Autodesk Inventor part; units mm, degrees
ref_plane "YZ Plane" through (0, 0, 0) normal (1, 0, 0) x (0, 1, 0)
ref_plane "XZ Plane" through (0, 0, 0) normal (0, 1, 0) x (-1, 0, 0)
ref_plane "XY Plane" through (0, 0, 0) normal (0, 0, 1) x (1, 0, 0)
sketch "Skizze3" plane through (0, 0, 0) normal (1, 0, 0) x (0, 1, 0)
  line L0 (0, 60) -> (0, -10) construction
  line L1 (-35, 0) -> (35, 0) construction
  line L2 (25, 0) -> (25, 22.5) construction
  line L3 (25, 50) -> (-25, 50)
  line L4 (-25, 50) -> (-25, 26)
  line L5 (11.1, 0) -> (11.1, 26) construction
  line L6 (11.1, 26) -> (-11.1, 26) construction
  line L7 (-11.1, 26) -> (-11.1, 0) construction
  line L8 (11.1, 22.5) -> (25, 22.5)
  line L9 (11.1, 22.5) -> (11.1, 26)
  line L10 (11.1, 26) -> (-25, 26)
  line L11 (-25, 26) -> (-25, 0) construction
  line L12 (25, 22.5) -> (25, 50)
  point P0 (0, 0)
  dimension "d8" = 100
  dimension "d9" = 50
  dimension "d10" = 52
  dimension "d11" = 22.2
  dimension "d13" = 45
revolve "Grundkörper" add sketch "Skizze3" angle 360 about axis through (0, 0, 0) along (0, 1, 0)
sketch "Skizze4" plane through (0, 0, 0) normal (1, 0, 0) x (0, 1, 0)
  line L0 (-25, 50) -> (25, 50) construction
  line L1 (0, 48) -> (0, -8) construction
  line L2 (-15, 50) -> (-15, 30)
  line L3 (-15, 30) -> (15, 30)
  line L4 (15, 30) -> (15, 50)
  line L5 (-15, 50) -> (15, 50)
  point P0 (0, 0)
  dimension "d17" = 30
  dimension "d18" = 20
extrude "Profil_Ausschnitt" cut sketch "Skizze4" along normal through all both and the other way through all
sketch "Skizze5" plane through (0, -25, 0) normal (0, -1, 0) x (1, 0, 0)
  circle A0 centre (0, 0) radius 50 construction
  line L0 (0, 70) -> (0, -70) construction
  line L1 (-40, 30) -> (40, 30) construction
  line L2 (0, 30) -> (0, 50) construction
  point P0 (0, 40)
hole "DIN7984_M8_Boh" at (0, -25, 40) direction (0, 1, 0) diameter 9 end up to surface counterbore diameter 15 counterbore depth 5.4
mirror "Spiegelung_DIN7984_M8_Boh" about plane through (0, 0, 0) normal (0, 1, 0) of "DIN7984_M8_Boh"
sketch "Skizze7" plane through (0, 0, 0) normal (1, 0, 0) x (0, 1, 0)
  line L0 (-35, 0) -> (35, 0) construction
  line L1 (11.1, -26) -> (11.1, 26) construction
  line L2 (11.1, 26) -> (-25, 26) construction
  line L3 (-11.1, 26) -> (-11.1, 27.5)
  line L4 (-11.1, 27.5) -> (-13.25, 27.5)
  line L5 (-13.25, 27.5) -> (-13.25, 26)
  line L6 (-11.1, 26) -> (-13.25, 26)
  point P0 (0, 0)
  dimension "d34" = 55
  dimension "d35" = 2.15
  dimension "d36" = 22.2
revolve "DIN472-52x2-Nut" cut sketch "Skizze7" angle 360 about axis through (0, 0, 0) along (0, 1, 0)
chamfer "Fase_Allgemein" distance 2 angle 45 4 edges at (0, -25, -50) (0, 25, -50) (0, -25, -26) (0, 25, -22.5)
chamfer "Fase2" distance 0.2 angle 45 1 edges at (0, 11.1, -22.5)
properties part number "200-30-ROCKER-BOGIE-BEARING-01" material "Aluminium 6061"
Design review of the part built by this model. Coordinates are the model's own, in mm. A direction names the side the tool comes from. Give positions to 0.01 mm unless a question says otherwise; leave off trailing zeros. Write each loop counter-clockwise with the first axis right and the second up, starting at its lowest first coordinate (ties: lowest second). Pieces come first, ordered by that corner, then holes. Notation, with made-up numbers: M 65.25,1.25 L 97.25,1.25 A22 cw 97.25,19.25 Z; hole C 89,32 d2. An arc over 180 degrees is marked long. Return JSON: item names as keys, results as strings. Group by question number.
Item 1: Take a section at C-C (x = 0). Count the separate pieces of the cut face and the enclosed holes in it, plus the area to 3 significant figures.
Item 2: Tool access review of faces 1 (the cylindrical face through (15.821, -18.193, -20.633)), 2 (the flat face through (-1, 15, 35)), 3 (the flat face through (-24.3, -11.1, 10.1)), 4 (the cylindrical face through (-0.33, 22.262, 32.507)): name each direction out of +Z, -Z, +X, -X, +Y, -Y from which nothing blocks a thin tool from reaching the whole face with its end or side.
Item 3: The part is to be moulded in two halves that separate along Z. For faces 5 (the conical face through (18.43, 24.87, 44.46)), 6 (the flat face through (-1, -15, 33)), 7 (the conical face through (25.504, -23.125, -5.663)), 8 (the cylindrical face through (-2.253, -22.262, 32.846)), say which applies: pulls with the +Z half, pulls with the -Z half, needs draft (parallel to the pull), parting line crosses it, or undercut.
Item 4: Clearance check with flat-ended pins moving along their axes: pin 1 Ø3 at (y, z) = (7.5, -26) entering from +X; pin 2 Ø14.5 at (x, z) = (0, 40) entering from +Y; pin 3 Ø2 at (x, y) = (29, 11) entering from +Z; pin 4 Ø6 at (x, z) = (38, 31) entering from +Y. State where each tip first meets the part, or that it passes through.
Item 5: Take a section at B-B (y = 7). Give the boundary of the cut face in (x, z).
Item 6: Wall thickness on line 1 along X through (y, z) = (-6, 0); line 2 along Y through (x, z) = (-13, 40); line 3 along Y through (x, z) = (-21, -18.5): over which ranges is each line inside the solid? List them lowest first.
Return value:
{
 "1": {"separate pieces": "4", "enclosed holes": "0", "area": "1,630 mm2"},
 "2": {"face 1": "-Y", "face 2": "+Z, +X, -X", "face 3": "none", "face 4": "+Y"},
 "3": {"face 5": "parting line crosses it", "face 6": "needs draft", "face 7": "undercut", "face 8": "undercut"},
 "4": {"pin 1": "stops at x = 43.59", "pin 2": "stops at y = 19.6", "pin 3": "stops at z = 30", "pin 4": "stops at y = 25"},
 "5": {"outline": "M -40,30 A50 ccw long 40,30 Z; hole C 0,0 d52"},
 "6": {"line 1": "x = -50 to -26, 26 to 50", "line 2": "y = -25 to -15, 15 to 25", "line 3": "y = -24.99 to 25"}
}
